Geometry: final body of the model. Coordinates: model frame, mm. Face numbers are marked on the shaded views. A direction names the side the tool comes from. Give positions to 0.01 mm unless a question says otherwise; leave off trailing zeros. Write each loop counter-clockwise with the first axis right and the second up, starting at its lowest first coordinate (ties: lowest second). Pieces come first, ordered by that corner, then holes. Notation, with made-up numbers: (-23.5, 88.25) - (24.5, 88.25) arc R13 ccw to (24.5, 107.25) - close; hole circle Ø6 at (-24.75, 42). An arc over 180 degrees is marked (long way). Return JSON: item names as keys, results as strings.
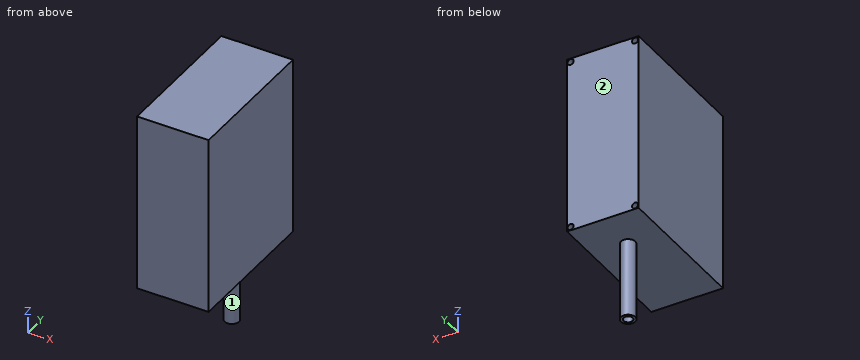
from build123d import *

# Parameters (mm, degrees)
SKETCH1_W           = 50
SKETCH1_H           = 100
BOSS_EXTRUDE1_DEPTH = 125
SKETCH2_R           = 5
BOSS_EXTRUDE2_DEPTH = 55
SKETCH3_R           = 2.1
CUT_EXTRUDE1_DEPTH  = 6
SKETCH4_R           = 3.2
CUT_EXTRUDE2_DEPTH  = 10


with BuildPart() as part:
    # Sketch1 → Boss-Extrude1 (new body)
    with BuildSketch(Plane.XY):
        Rectangle(SKETCH1_W, SKETCH1_H)
    extrude(amount=BOSS_EXTRUDE1_DEPTH)

    # Sketch2 → Boss-Extrude2 (add)
    with BuildSketch(Plane.XY):
        with Locations((0, 20)):
            Circle(SKETCH2_R)
    extrude(amount=-BOSS_EXTRUDE2_DEPTH)

    # Sketch3 → Cut-Extrude1 (cut)
    with BuildSketch(Plane(origin=(0, 50, 0), x_dir=(1, 0, 0), z_dir=(0, 1, 0))):
        with Locations(Location((-22.5, -2.5, 0), (0, 0, 270))):
            Circle(SKETCH3_R)
        with Locations(Location((22.5, -2.5, 0), (0, 0, 270))):
            Circle(SKETCH3_R)
        with Locations(Location((22.5, -122.5, 0), (0, 0, 270))):
            Circle(SKETCH3_R)
        with Locations(Location((-22.5, -122.5, 0), (0, 0, 270))):
            Circle(SKETCH3_R)
    extrude(amount=-CUT_EXTRUDE1_DEPTH, mode=Mode.SUBTRACT)

    # Sketch4 → Cut-Extrude2 (cut)
    with BuildSketch(Plane(origin=(0, 0, -55), x_dir=(-1, 0, 0), z_dir=(0, 0, -1))):
        with Locations((0, 20)):
            Circle(SKETCH4_R)
    extrude(amount=-CUT_EXTRUDE2_DEPTH, mode=Mode.SUBTRACT)


solid = part.part
Q1. Material intervals for probe 1 along X at (y, z) = (47.05, 2.5); probe 2 along X at (y, z) = (47, 122); probe 3 along Z at (x, y) = (1, -27.5), sorted ascending. Write a range as [from, to].
Answer key:
{"probe 1": "x = [-25, -24.6], [-20.4, 20.4], [24.6, 25]", "probe 2": "x = [-25, -24.54], [-20.46, 20.46], [24.54, 25]", "probe 3": "z = [0, 125]"}
Q2. Section query A-A, the plane x = 22.5. Return the cut outline in (y, z).
Answer key:
{"outline": "(-50, 0) - (50, 0) - (50, 0.4) - (44, 0.4) - (44, 4.6) - (50, 4.6) - (50, 120.4) - (44, 120.4) - (44, 124.6) - (50, 124.6) - (50, 125) - (-50, 125) - close"}
Q3. Section query D-D, the plane x = -10. Return the cut outline in (y, z), plus the area to 3 significant figures.
Answer key:
{"outline": "(-50, 0) - (50, 0) - (50, 125) - (-50, 125) - close", "area": "12,500 mm^2"}
Q4. Section query C-C, the plane z = -30. Return the cut outline in (x, y).
Answer key:
{"outline": "circle Ø10 at (0, 20)"}
Q5. Section query B-B, the plane y = 20. Return the cut outline in (x, z).
Answer key:
{"outline": "(-25, 0) - (-5, 0) - (-5, -55) - (-3.2, -55) - (-3.2, -45) - (3.2, -45) - (3.2, -55) - (5, -55) - (5, 0) - (25, 0) - (25, 125) - (-25, 125) - close"}
Q6. Set-up query: the marked faces 1 and 2. Return all of +Z, -Z, +X, -X, +Y, -Y with unobstructed straight access to the full face (end or side cutting, diameter ignored); none if empty.
Answer key:
{"face 1": "-Z", "face 2": "+Z, -Z, +X, -X, +Y"}
Q7. Pin query (flat end, axial travel): P1, Ø5, axis at x = 6.5, y = -22, coming from the -Z side; P2, Ø2.5, axis at x = -22.5, z = 122.5, coming from the +Y side. Return the tip coordinate at first contact, or that it passes through.
Answer key:
{"P1": "stops at z = 0", "P2": "stops at y = 44"}
